from build123d import *

# Parameters (mm, degrees)
F2_R     = 2.75
F2_R_2   = 3.25
F2_R_3   = 12.5
F3_DEPTH = 3
F4_SIZE  = 2


with BuildPart() as f1:
    # F0 (on Right) → F1 (revolve)
    with BuildSketch(Plane.YZ):
        Polygon((0, 12.5), (0, 42.5), (-37, 42.5), (-37, 37.75), (-22, 37.75), (-22, 21.1), (-5, 21.1), (-5, 12.5), align=None)
    revolve(axis=Axis((0, -4.4609829783, 0), (0, 1, 0)))

    # F2 (on Front) → F3 (join)
    with BuildSketch(Plane.XZ):
        Polygon((42.5, 0), (42.5, 42.5), (-42.5, 42.5), (-42.5, 0), (-42.5, -42.5), (-42.5, -60), (42.5, -60), (42.5, -42.5), align=None)
        with Locations((-37, -37)):
            Circle(F2_R, mode=Mode.SUBTRACT)
        with Locations((-28.2, -46.052)):
            Circle(F2_R_2, mode=Mode.SUBTRACT)
        with Locations((14.3, -46.052)):
            Circle(F2_R_2, mode=Mode.SUBTRACT)
        with Locations((37, -37)):
            Circle(F2_R, mode=Mode.SUBTRACT)
        with Locations((-37, 37)):
            Circle(F2_R, mode=Mode.SUBTRACT)
        Circle(F2_R_3, mode=Mode.SUBTRACT)
        with Locations((37, 37)):
            Circle(F2_R, mode=Mode.SUBTRACT)
    extrude(amount=F3_DEPTH)

    # F4
    f4_edges = [f1.edges().sort_by_distance(p)[0] for p in [
        (42.5, -1.5, 42.5),
        (-42.5, -1.5, 42.5),
        (42.5, -1.5, -60),
        (-42.5, -1.5, -60),
        (0, -22, -21.1),
        (0, -37, -37.75),
    ]]
    chamfer(f4_edges, length=F4_SIZE)


solid = f1.part
Design review of the part built by this model. Coordinates are the model's own, in mm. A direction names the side the tool comes from. Coordinates: 2 decimals unless noted, no trailing zeros. Loops run counter-clockwise (first coordinate to the right, second up) from the corner with the lowest first, then second, coordinate; pieces in that order, holes last. Notation, with made-up numbers: (47.25, -26.5) -> (66.25, -26.5) arc R25 ccw to (66.25, -14.5) -> close; hole circle Ø1 at (15, 44). An arc over 180 degrees is marked (long way). Use a Markdown table: item, result. Add a question column.
Item 1: We need section B-B, the plane z = -51. Write out the cut boundary in (x, y), and give its area (3 significant figures).
Item 2: We need section C-C, the plane y = -31.5. Write out the cut boundary in (x, z).
Item 3: The part is to be moulded in two halves that separate along Z. For faces 4 (the flat face through (-10, 0, -8)), 5 (the cylindrical face through (-39.027, -1.479, 38.859)), 6 (the flat face through (1, -1, 42.5)), say which applies: +Z half, -Z half, draft (parallel to the pull), parting line (faces both ways), or undercut.
Item 4: We need section A-A, the plane y = -11.5. Write out the cut boundary in (x, z), and give its area (3 significant figures).
Item 5: Wall thickness on L1, parallel to Z at x = 37, y = -2.35; L2, parallel to Z at x = 0, y = -1.55; L3, parallel to X at y = -25, z = 0: over which ranges is each line inside the solid? List them lowest first. Write a range as from..to.
Item 6: Machinability: for faces 1 (the flat face through (32, -3, 34)), 2 (the flat face through (-32, -3, 34)), 3 (the cylindrical face through (-25.861, -20.238, -33.727)), which of the approach directions +Z, -Z, +X, -X, +Y, -Y give a long, thin tool a straight path to every point of the face, cutting with its end or side? Answer none if there is none.
Item 7: Clearance check with flat-ended pins moving along their axes: P1, Ø21, axis at x = 6.5, z = -1.5, coming from the -Y side; P2, Ø5, axis at x = 37, z = 37, coming from the -Y side; P3, Ø1.5, axis at x = 18.5, y = -28.5, coming from the -Z side; P4, Ø6, axis at x = -32.5, y = -26, coming from the -Z side. State where each tip first meets the part, or that it passes through.
Numbers:
| question | item | result |
|---|---|---|
| 1 | outline | (-42.5, -3) -> (42.5, -3) -> (42.5, 0) -> (-42.5, 0) -> close |
| 1 | area | 255 mm^2 |
| 2 | outline | circle Ø85 at (0, 0); hole circle Ø75.5 at (0, 0) |
| 3 | face 4 | draft |
| 3 | face 5 | undercut |
| 3 | face 6 | +Z half |
| 4 | outline | circle Ø85 at (0, 0); hole circle Ø42.2 at (0, 0) |
| 4 | area | 4,280 mm^2 |
| 5 | L1 | z = -60..-39.75, -34.25..34.25, 39.75..42.5 |
| 5 | L2 | z = -60..-12.5, 12.5..42.5 |
| 5 | L3 | x = -42.5..-37.75, 37.75..42.5 |
| 6 | face 1 | +Z, +X, -Y |
| 6 | face 2 | +Z, -X, -Y |
| 6 | face 3 | -Y |
| 7 | P1 | stops at y = -5 |
| 7 | P2 | passes through |
| 7 | P3 | stops at z = -38.62 |
| 7 | P4 | stops at z = -30.59 |
